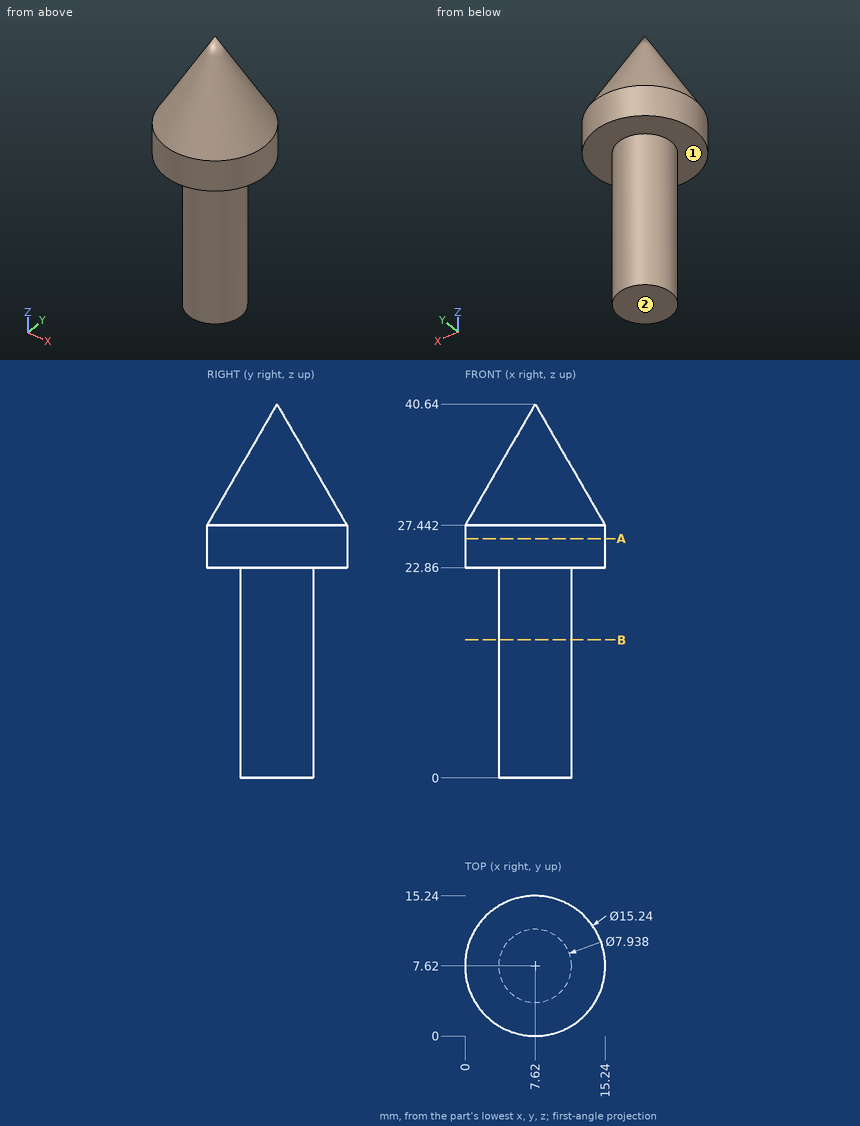
Input: dimensioned drawing with shaded views. Units: mm. Origin: part minimum x, y, z. A direction names the side the tool comes from. Coordinates: 2 decimals unless noted, no trailing zeros. Loops run counter-clockwise (first coordinate to the right, second up) from the corner with the lowest first, then second, coordinate; pieces in that order, holes last. Notation, with made-up numbers: (-17, 3) -> (33, 3) arc R29 ccw to (33, 23) -> close; hole circle Ø2 at (-8, -25.75). An arc over 180 degrees is marked (long way). Use a Markdown table: item, result. Add a question column.
(1) Pin query (flat end, axial travel): pin 1 Ø8 at (y, z) = (12, 35) entering from -X (1 decimal); pin 2 Ø1 at (x, y) = (6, 13.5) entering from +Z (1 decimal); pin 3 Ø8 at (x, z) = (9.5, 8) entering from -Y; pin 4 Ø1 at (x, z) = (12.5, 7.5) entering from +Y. Return the tip coordinate at first contact, or that it passes through.
(2) Line query: line 1 along X through (y, z) = (7.25, 26); line 2 along Z through (x, y) = (10, 1) (1 decimal); line 3 along X through (y, z) = (7.75, 9). Output: solid intervals per line, ascending.
(3) Section query B-B, the plane z = 15. Return loops of the section in (x, y), plus the area to 3 significant figures.
(4) Section query A-A, the plane z = 26. Return loops of the section in (x, y), plus the area to 3 significant figures.
(5) Access query for the marked faces 1 and 2. Directions: +Z, -Z, +X, -X, +Y, -Y. A direction counts if a zero-diameter tool reaches every point of the face in a straight line with its end or side. Return the directions, or none.
Answer:
| question | item | result |
|---|---|---|
| 1 | pin 1 | stops at x = 2.9 |
| 1 | pin 2 | stops at z = 30.9 |
| 1 | pin 3 | stops at y = 3.65 |
| 1 | pin 4 | passes through |
| 2 | line 1 | x = 0.01 to 15.23 |
| 2 | line 2 | z = 22.9 to 28.5 |
| 2 | line 3 | x = 3.65 to 11.59 |
| 3 | outline | circle Ø7.94 at (7.62, 7.62) |
| 3 | area | 49.5 mm^2 |
| 4 | outline | circle Ø15.24 at (7.62, 7.62) |
| 4 | area | 182 mm^2 |
| 5 | face 1 | -Z |
| 5 | face 2 | -Z, +X, -X, +Y, -Y |
